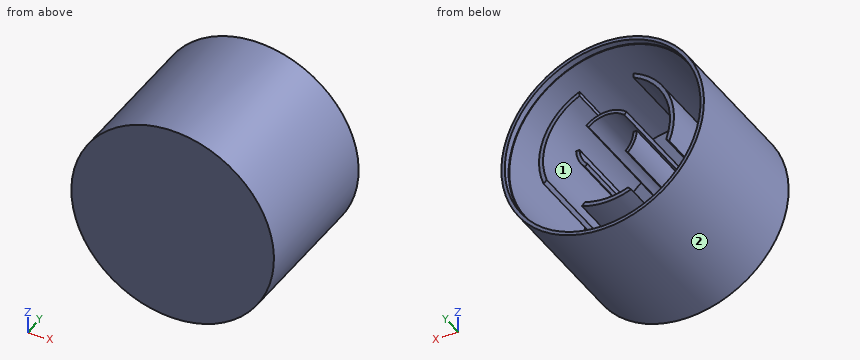
from build123d import *

# Parameters (mm, degrees)
SKETCH1_R           = 75
BOSS_EXTRUDE1_DEPTH = 110
SKETCH2_R           = 72
CUT_EXTRUDE1_DEPTH  = 100
SKETCH3_R           = 72.5
CUT_EXTRUDE2_DEPTH  = 5
SKETCH8_R           = 50
SKETCH8_R_2         = 47
BOSS_EXTRUDE4_DEPTH = 95
SKETCH10_R          = 22.5
SKETCH10_R_2        = 20
BOSS_EXTRUDE5_DEPTH = 95
CUT_EXTRUDE3_START  = -95
SKETCH11_W          = 20
SKETCH11_H          = 27.4
CUT_EXTRUDE3_DEPTH  = 95


with BuildPart() as part:
    # Sketch1 → Boss-Extrude1 (new body)
    with BuildSketch(Plane(origin=(0, 0, 0), x_dir=(1, 0, 0), z_dir=(0, 1, 0))):
        with Locations(Location((0, 0, 0), (0, 0, 90))):
            Circle(SKETCH1_R)
    extrude(amount=BOSS_EXTRUDE1_DEPTH)

    # Sketch2 → Cut-Extrude1 (cut)
    with BuildSketch(Plane(origin=(0, 110, 0), x_dir=(1, 0, 0), z_dir=(0, 1, 0))):
        with Locations(Location((0, 0, 0), (0, 0, 270))):
            Circle(SKETCH2_R)
    extrude(amount=-CUT_EXTRUDE1_DEPTH, mode=Mode.SUBTRACT)

    # Sketch3 → Cut-Extrude2 (cut)
    with BuildSketch(Plane(origin=(0, 110, 0), x_dir=(1, 0, 0), z_dir=(0, 1, 0))):
        with Locations(Location((0, 0, 0), (0, 0, 270))):
            Circle(SKETCH3_R)
    extrude(amount=-CUT_EXTRUDE2_DEPTH, mode=Mode.SUBTRACT)

    # Sketch8 → Boss-Extrude4 (add)
    with BuildSketch(Plane(origin=(0, 10, 0), x_dir=(1, 0, 0), z_dir=(0, 1, 0))):
        with Locations(Location((0, 0, 0), (0, 0, 270))):
            Circle(SKETCH8_R)
        with Locations(Location((0, 0, 0), (0, 0, 270))):
            Circle(SKETCH8_R_2, mode=Mode.SUBTRACT)
    extrude(amount=BOSS_EXTRUDE4_DEPTH)

    # Sketch10 → Boss-Extrude5 (add)
    with BuildSketch(Plane(origin=(0, 10, 0), x_dir=(1, 0, 0), z_dir=(0, 1, 0))):
        with Locations(Location((0, 0, 0), (0, 0, 270))):
            Circle(SKETCH10_R)
        with Locations(Location((0, 0, 0), (0, 0, 270))):
            Circle(SKETCH10_R_2, mode=Mode.SUBTRACT)
    extrude(amount=BOSS_EXTRUDE5_DEPTH)

    # Sketch11 → Cut-Extrude3 (cut)
    with BuildSketch(Plane(origin=(0, 105, 0), x_dir=(1, 0, 0), z_dir=(0, 1, 0)).offset(CUT_EXTRUDE3_START)):
        with Locations((-10, -36.3)):
            Rectangle(SKETCH11_W, SKETCH11_H)
        with Locations((10, -36.3)):
            Rectangle(SKETCH11_W, SKETCH11_H)
        Polygon((-35.352400393, 35.358277481), (-15.986116357, 15.988773936), (-15.984553545, 15.990430632), (-2.254814273, 30.544962608), (-21.21026477, 49.500413105), align=None)
        Polygon((-49.494536017, 21.216141857), (-29.714292817, 1.435898657), (-15.986116357, 15.988773936), (-35.352400393, 35.358277481), align=None)
        Polygon((2.486026551, 30.767534041), (15.99775062, 15.995091549), (35.358277481, 35.352400393), (21.217317324, 49.495711386), align=None)
        Polygon((35.358277481, 35.352400393), (15.99775062, 15.995091549), (29.509474689, 1.222649056), (49.499237638, 21.209089401), align=None)
        with BuildLine():
            ThreePointArc((-13.25433726, -14.977401103), (-18.428729118, -7.770581901), (-19.97668921, 0.96534356))
            Line((-19.97668921, 0.96534356), (-22.473775362, 1.086011505))
            ThreePointArc((-22.473775362, 1.086011505), (-20.732320258, -8.741904639), (-14.911129417, -16.849576241))
            Line((-14.911129417, -16.849576241), (-13.25433726, -14.977401103))
        make_face()
        with BuildLine():
            ThreePointArc((20, 0), (18.235771785, -8.213198366), (13.25433726, -14.977401103))
            Line((13.25433726, -14.977401103), (14.911129417, -16.849576241))
            ThreePointArc((14.911129417, -16.849576241), (20.515243258, -9.239848162), (22.5, 0))
            ThreePointArc((22.5, 0), (22.495177624, 0.46581504), (22.480712564, 0.931430406))
            Line((22.480712564, 0.931430406), (19.982855613, 0.827938139))
            ThreePointArc((19.982855613, 0.827938139), (19.995713444, 0.414057814), (20, 0))
        make_face()
        with BuildLine():
            Line((-15.908580177, 15.911224866), (-14.140960157, 14.143310992))
            ThreePointArc((-14.140960157, 14.143310992), (0.001662291, 19.999999931), (14.143310992, 14.140960157))
            Line((14.143310992, 14.140960157), (15.911224866, 15.908580177))
            ThreePointArc((15.911224866, 15.908580177), (0.001870078, 22.499999922), (-15.908580177, 15.911224866))
        make_face()
    extrude(amount=CUT_EXTRUDE3_DEPTH, mode=Mode.SUBTRACT)


solid = part.part
Design review of the part built by this model. Coordinates are the model's own, in mm. Face numbers are marked on the shaded views. A direction names the side the tool comes from. Round coordinates to 2 decimals unless told otherwise and drop trailing zeros. Order: outer loops, then holes, each group sorted by start corner. A loop starts at its lowest first (then second) coordinate and runs counter-clockwise, first axis right, second up.
1) For L1, parallel to X at y = 37, z = 0; L2, parallel to Z at x = -40, y = 80.5; L3, parallel to X at y = 75, z = 5, list the stretches that pass through material, from the lowest coordinate up.
The answers:
L1: x = -75 to -72, -50 to -47, 47 to 50, 72 to 75
L2: z = -63.44 to -59.87, 24.68 to 30, 59.87 to 63.44
L3: x = -74.83 to -71.83, -49.75 to -46.73, 46.73 to 49.75, 71.83 to 74.83
2) Machinability: for the marked faces 1 and 2, which of the approach directions +Z, -Z, +X, -X, +Y, -Y give a long, thin tool a straight path to every point of the face, cutting with its end or side? Answer none if there is none.
The answers:
face 1: +Y
face 2: +Y, -Y
3) Consider section A-A (y = 63.5). State the section outline as (x, z) points.
The answers:
outline: circle Ø150 at (0, 0); (-46.54, -18.27) - (-44.22, -15.94) arc R47 cw to (-20, 42.53) - (-20, 45.83) arc R50 ccw to start; (-22.47, -1.09) arc R22.5 ccw to (-15.91, -15.91) - (-14.14, -14.14) arc R20 cw to (-19.98, -0.97) - close; (-18.26, -46.55) arc R50 ccw to (18.27, -46.54) - (15.94, -44.22) arc R47 cw to (-15.93, -44.22) - close; (-14.91, 16.85) - (-13.25, 14.98) arc R20 cw to (13.25, 14.98) - (14.91, 16.85) arc R22.5 ccw to start; (14.14, -14.14) - (15.91, -15.91) arc R22.5 ccw to (22.48, -0.93) - (19.98, -0.83) arc R20 cw to start; (20, 42.53) arc R47 cw to (44.22, -15.93) - (46.55, -18.26) arc R50 ccw to (20, 45.83) - close; hole circle Ø144 at (0, 0)
4) Consider section D-D (x = -52). State the section outline as (y, z) points.
The answers:
outline: (0, -54.05) - (110, -54.05) - (110, -50.52) - (105, -50.52) - (105, -49.8) - (10, -49.8) - (10, 49.8) - (105, 49.8) - (105, 50.52) - (110, 50.52) - (110, 54.05) - (0, 54.05) - close
5) Clearance check with flat-ended pins moving along their axes: pin 1 Ø9 at (x, z) = (37.5, 6.5) entering from +Y; pin 2 Ø1.5 at (x, y) = (-50.5, 17.5) entering from -Z; pin 3 Ø1 at (x, y) = (44, 88.5) entering from -Z. State where each tip first meets the part, or that it passes through.
The answers:
pin 1: stops at y = 10
pin 2: stops at z = -56.12
pin 3: stops at z = -61.1
6) Consider section B-B (x = 0). State the section outline as (y, z) points.
The answers:
outline: (0, -75) - (110, -75) - (110, -72.5) - (105, -72.5) - (105, -72) - (10, -72) - (10, -50) - (105, -50) - (105, -47) - (10, -47) - (10, 20) - (105, 20) - (105, 22.5) - (10, 22.5) - (10, 72) - (105, 72) - (105, 72.5) - (110, 72.5) - (110, 75) - (0, 75) - close
7) Consider section C-C (z = 58.5). State the section outline as (x, y) points.
The answers:
outline: (-46.93, 0) - (46.93, 0) - (46.93, 110) - (42.83, 110) - (42.83, 105) - (41.97, 105) - (41.97, 10) - (-41.97, 10) - (-41.97, 105) - (-42.83, 105) - (-42.83, 110) - (-46.93, 110) - close
